Geometry: final body of the model. Coordinates: model frame, mm. A direction names the side the tool comes from. Coordinates: 2 decimals unless noted, no trailing zeros. Loops run counter-clockwise (first coordinate to the right, second up) from the corner with the lowest first, then second, coordinate; pieces in that order, holes last. Notation, with made-up numbers: (-4, 2.5) - (7, 2.5) arc R22 cw to (7, 19.5) - close; hole circle Ø8 at (72, -18). An arc over 180 degrees is marked (long way). Answer in a Markdown table with one row per item.
from build123d import *

# Parameters (mm, degrees)
SKIZZE1_R                       = 6
AUFSATZ_LINEAR_AUSTRAGEN1_DEPTH = 3.5
SKIZZE1_3_R                     = 3.5
SCHNITT_LINEAR_AUSTRAGEN1_DEPTH = 2.5
SKIZZE1_4_R                     = 2.5
SCHNITT_LINEAR_AUSTRAGEN3_DEPTH = 4.5
SCHNITT_LINEAR_START            = -1
SKIZZE1_5_OUTSIDE_W             = 17.466
SKIZZE1_5_OUTSIDE_H             = 17.466
SKIZZE1_5_OUTSIDE_W_2           = 8
SKIZZE1_5_OUTSIDE_H_2           = 8
SCHNITT_LINEAR_AUSTRAGEN4_DEPTH = 3.5


with BuildPart() as part:
    # Skizze1 → Aufsatz-Linear austragen1 (new body)
    with BuildSketch(Plane.XY):
        Circle(SKIZZE1_R)
    extrude(amount=-AUFSATZ_LINEAR_AUSTRAGEN1_DEPTH)

    # Skizze1<3> → Schnitt-Linear austragen1 (cut)
    with BuildSketch(Plane.XY):
        Circle(SKIZZE1_3_R)
    extrude(amount=-SCHNITT_LINEAR_AUSTRAGEN1_DEPTH, mode=Mode.SUBTRACT)

    # Skizze1<4> → Schnitt-Linear austragen3 (cut, through all)
    with BuildSketch(Plane.XY):
        Circle(SKIZZE1_4_R)
    extrude(amount=-SCHNITT_LINEAR_AUSTRAGEN3_DEPTH, mode=Mode.SUBTRACT)

    # Skizze1<5> outside → Schnitt-Linear austragen4 (cut, through all)
    with BuildSketch(Plane.XY.offset(SCHNITT_LINEAR_START)):
        Rectangle(SKIZZE1_5_OUTSIDE_W, SKIZZE1_5_OUTSIDE_H)
        Rectangle(SKIZZE1_5_OUTSIDE_W_2, SKIZZE1_5_OUTSIDE_H_2, mode=Mode.SUBTRACT)
    extrude(amount=-SCHNITT_LINEAR_AUSTRAGEN4_DEPTH, mode=Mode.SUBTRACT)


solid = part.part
(1) Cut plane C-C on z = -1.45. Output: boundary loops of the cut face in (x, y).
Verdict:
| item | result |
|---|---|
| outline | (-4, -4) - (4, -4) - (4, 4) - (-4, 4) - close; hole circle Ø7 at (0, 0) |
(2) First-contact query: pin 1 Ø1.2 at (y, z) = (-1.5, -1.5) entering from +X; pin 2 Ø3.5 at (x, y) = (0, 1) entering from +Z; pin 3 Ø2 at (x, z) = (-1, -1.5) entering from -Y; pin 4 Ø4 at (x, y) = (0, 0) entering from -Z. Flat tips, straight axial feed; report the tip coordinate or a pass-through.
Verdict:
| item | result |
|---|---|
| pin 1 | stops at x = 5.89 |
| pin 2 | stops at z = -2.5 |
| pin 3 | stops at y = -6 |
| pin 4 | passes through |
(3) Access query for faces 1 (the face through (0, 4, -2)), 2 (the face through (4, 0, -2)), 3 (the face through (-4, 0, -2)), 4 (the face through (3.233, -1.341, -1.232)), 5 (the face through (0, -4, -2)). Directions: +Z, -Z, +X, -X, +Y, -Y. A direction counts if a zero-diameter tool reaches every point of the face in a straight line with its end or side. Return the directions, or none.
Verdict:
| item | result |
|---|---|
| face 1 | -Z, +X, -X, +Y |
| face 2 | -Z, +X, +Y, -Y |
| face 3 | -Z, -X, +Y, -Y |
| face 4 | +Z |
| face 5 | -Z, +X, -X, -Y |
(4) Cut plane A-A on x = 0. Output: boundary loops of the cut face in (y, z), then the cut area to 3 significant figures.
Verdict:
| item | result |
|---|---|
| outline | (-6, -1) - (-4, -1) - (-4, -3.5) - (-2.5, -3.5) - (-2.5, -2.5) - (-3.5, -2.5) - (-3.5, 0) - (-6, 0) - close; (2.5, -3.5) - (4, -3.5) - (4, -1) - (6, -1) - (6, 0) - (3.5, 0) - (3.5, -2.5) - (2.5, -2.5) - close |
| area | 9.50 mm² |
(5) Cut plane D-D on z = -3.3. Output: boundary loops of the cut face in (x, y), then the cut area to 3 significant figures.
Verdict:
| item | result |
|---|---|
| outline | (-4, -4) - (4, -4) - (4, 4) - (-4, 4) - close; hole circle Ø5 at (0, 0) |
| area | 44.4 mm² |
(6) Ray query, probe 1 along Y at (x, z) = (0, -0.6); probe 2 along Y at (x, z) = (0, -2.85); probe 3 along Z at (x, y) = (-2, 4.5). Return the intervals inside material, ascending.
Verdict:
| item | result |
|---|---|
| probe 1 | y = -6 to -3.5, 3.5 to 6 |
| probe 2 | y = -4 to -2.5, 2.5 to 4 |
| probe 3 | z = -1 to 0 |
